from build123d import *

# Parameters (mm, degrees)
SKETCH1_W           = 76.2
SKETCH1_H           = 177.8
BOSS_EXTRUDE1_DEPTH = 63.5
SKETCH2_R           = 38.1
BOSS_EXTRUDE2_DEPTH = 63.5
SKETCH4_R           = 13.97
CUT_EXTRUDE1_DEPTH  = 48.26
FILLET2_R           = 25.4


with BuildPart() as part:
    # Sketch1 → Boss-Extrude1 (new body)
    with BuildSketch(Plane.XY):
        Rectangle(SKETCH1_W, SKETCH1_H)
    extrude(amount=BOSS_EXTRUDE1_DEPTH)

    # Sketch2 → Boss-Extrude2 (add, through all)
    with BuildSketch(Plane.XY):
        with Locations((0, -88.9)):
            Circle(SKETCH2_R)
    extrude(amount=BOSS_EXTRUDE2_DEPTH)

    # Sketch4 → Cut-Extrude1 (cut)
    with BuildSketch(Plane.XY):
        with Locations(Location((0, -88.9, 0), (0, 0, 180))):
            Circle(SKETCH4_R)
    extrude(amount=CUT_EXTRUDE1_DEPTH, mode=Mode.SUBTRACT)

    # Fillet2
    fillet2_edges = [part.edges().sort_by_distance(p)[0] for p in [
        (0, 88.9, 0),
        (-38.1, 88.9, 31.75),
        (38.1, 88.9, 31.75),
        (0, 88.9, 63.5),
    ]]
    fillet(fillet2_edges, radius=FILLET2_R)

    # Sketch5 → Cut-Revolve4 (revolve, cut)
    with BuildSketch(Plane(origin=(0, 0, 0), x_dir=(0, 0, -1), z_dir=(1, 0, 0))):
        with BuildLine():
            Line((-31.75, 53.823933451), (-31.75, 94.463933451))
            ThreePointArc((-31.75, 94.463933451), (-52.07, 74.143933451), (-31.75, 53.823933451))
        make_face()
    revolve(axis=Axis((0, 53.823933451, 31.75), (0, 1, 0)), mode=Mode.SUBTRACT)


solid = part.part
Model file for the job. Use its own axes, mm. A direction names the side the tool comes from. Coordinates: 2 decimals unless noted, no trailing zeros. Write each loop counter-clockwise with the first axis right and the second up, starting at its lowest first coordinate (ties: lowest second). Pieces come first, ordered by that corner, then holes. Notation, with made-up numbers: (72.5, -1.75) -> (107.5, -1.75) arc R25 ccw to (107.5, 11.25) -> close; hole circle Ø9 at (-24.75, 38). An arc over 180 degrees is marked (long way). One line per item, written item: value. Start each with the question number.
1) Which spindle directions (+Z, -Z, +X, -X, +Y, -Y) get a long thin tool onto all of the face, cutting with end or side? Do faces 1 (the face through (-7.51, -100.68, 23.79)), 2 (the face through (-0.84, -126.99, 31.31)). Say none if no direction does.
2) Slice it at C-C on x = -10. Write the cut outline in (y, z).
3) Slice it at D-D on y = -82. Write the cut outline in (x, z).
4) Slice it at B-B on y = 74. Write the cut outline in (x, z).
5) Slice it at A-A on z = 8. Write the cut outline in (x, y), then the cut area to 3 significant figures.
6) Probe probe 1 along X at (y, z) = (-88, 11); probe 2 along X at (y, z) = (-88.9, 21); probe 3 along Z at (x, y) = (-5.5, -95). List the from-to ranges inside material, lowest first.
7) Pull direction Y, two halves, no side cores. Call faces 3 (the face through (0.533, 77.839, 4.435)), 4 (the face through (0, -89, 48.26)), 5 (the face through (-38.1, -14, 31)): +Y half, -Y half, draft (parallel to the pull), parting line (faces both ways), or undercut.
8) Flat gauge pins, fed straight in: pin 1 Ø2 at (x, z) = (20, 17.5) entering from -Y; pin 2 Ø2 at (x, z) = (9.5, 31.5) entering from +Y; pin 3 Ø3 at (x, z) = (13, 34) entering from +Y. Where does each tip first touch, or does it go through?
Answers follow:
1. face 1: -Z
1. face 2: +Z, -Z, -Y
2. outline: (-125.66, 0) -> (-98.66, 0) -> (-98.66, 48.26) -> (-79.14, 48.26) -> (-79.14, 0) -> (63.5, 0) arc R25.4 ccw to (88.61, 21.57) arc R17.69 cw (long way) to (88.61, 41.93) arc R25.4 ccw to (63.5, 63.5) -> (-125.66, 63.5) -> close
3. outline: (-38.1, 0) -> (-12.15, 0) -> (-12.15, 48.26) -> (12.15, 48.26) -> (12.15, 0) -> (38.1, 0) -> (38.1, 63.5) -> (-38.1, 63.5) -> close
4. outline: (-35.83, 2.27) -> (35.83, 2.27) -> (35.83, 61.23) -> (-35.83, 61.23) -> close; hole circle Ø40.64 at (0, 31.75)
5. outline: (-38.1, -88.9) arc R38.1 ccw to (38.1, -88.9) -> (38.1, 63.5) arc R25.4 ccw to (30.1, 82) -> (-30.1, 82) arc R25.4 ccw to (-38.1, 63.5) -> close; hole circle Ø27.94 at (0, -88.9)
5. area: 14,600 mm2
6. probe 1: -38.1 to -13.94, 13.94 to 38.1
6. probe 2: -38.1 to -13.97, 13.97 to 38.1
6. probe 3: 48.26 to 63.5
7. face 3: +Y half
7. face 4: undercut
7. face 5: draft
8. pin 1: y = -121.92
8. pin 2: y = 56.75
8. pin 3: y = 88.89
